from build123d import *

# Parameters (mm, degrees)
CROQUIS1_R              = 1.5
SALIENTE_EXTRUIR1_DEPTH = 3
CROQUIS2_W              = 31.2
CROQUIS2_H              = 31.2
CROQUIS2_W_2            = 28.2
CROQUIS2_H_2            = 28.2
SALIENTE_EXTRUIR2_DEPTH = 9.5
CROQUIS4_W              = 28.2
CROQUIS4_H              = 28.2
CROQUIS4_W_2            = 26.2
CROQUIS4_H_2            = 26.2
SALIENTE_EXTRUIR3_DEPTH = 3
CORTAR_EXTRUIR1_REACH   = 69.732
CROQUIS8_W              = 7.2
CROQUIS8_H              = 1
CORTAR_EXTRUIR2_START   = -9.5
CROQUIS9_W              = 5.627722912
CROQUIS9_H              = 14.2
CORTAR_EXTRUIR2_DEPTH   = 9.5
CROQUIS10_W             = 2.5
CROQUIS10_H             = 31.2
SALIENTE_EXTRUIR4_DEPTH = 1


with BuildPart() as part:
    # Croquis1 → Saliente-Extruir1 (new body)
    with BuildSketch(Plane.XY):
        with BuildLine():
            Line((-52.197309417, 4.461883408), (-50.197309417, 4.461883408))
            Line((-50.197309417, 4.461883408), (-44.197309417, 8.461883408))
            Line((-44.197309417, 8.461883408), (-44.197309417, 24.461883408))
            Line((-44.197309417, 24.461883408), (-50.197309417, 28.461883408))
            Line((-50.197309417, 28.461883408), (-52.197309417, 28.461883408))
            ThreePointArc((-52.197309417, 28.461883408), (-56.197309417, 32.461883408), (-52.197309417, 36.461883408))
            Line((-52.197309417, 36.461883408), (-5.197309417, 36.461883408))
            ThreePointArc((-5.197309417, 36.461883408), (-3.075989073, 35.583203752), (-2.197309417, 33.461883408))
            Line((-2.197309417, 33.461883408), (-2.197309417, 26.567434684))
            ThreePointArc((-2.197309417, 26.567434684), (-2.552285621, 25.151860907), (-3.533208828, 24.071283801))
            Line((-3.533208828, 24.071283801), (-7.361410006, 21.519149682))
            ThreePointArc((-7.361410006, 21.519149682), (-8.342333213, 20.438572576), (-8.697309417, 19.022998799))
            Line((-8.697309417, 19.022998799), (-8.697309417, 13.900768017))
            ThreePointArc((-8.697309417, 13.900768017), (-8.342333213, 12.48519424), (-7.361410006, 11.404617134))
            Line((-7.361410006, 11.404617134), (-3.533208828, 8.852483016))
            ThreePointArc((-3.533208828, 8.852483016), (-2.552285621, 7.771905909), (-2.197309417, 6.356332133))
            Line((-2.197309417, 6.356332133), (-2.197309417, -0.538116592))
            ThreePointArc((-2.197309417, -0.538116592), (-3.075989073, -2.659436935), (-5.197309417, -3.538116592))
            Line((-5.197309417, -3.538116592), (-52.197309417, -3.538116592))
            ThreePointArc((-52.197309417, -3.538116592), (-56.197309417, 0.461883408), (-52.197309417, 4.461883408))
        make_face()
        with Locations((-6.697309417, 32.461883408)):
            Circle(CROQUIS1_R, mode=Mode.SUBTRACT)
        with Locations((-52.197309417, 0.461883408)):
            Circle(CROQUIS1_R, mode=Mode.SUBTRACT)
        with Locations((-6.697309417, 0.461883408)):
            Circle(CROQUIS1_R, mode=Mode.SUBTRACT)
        with Locations((-52.197309417, 32.461883408)):
            Circle(CROQUIS1_R, mode=Mode.SUBTRACT)
    extrude(amount=SALIENTE_EXTRUIR1_DEPTH)

    # Croquis2 → Saliente-Extruir2 (add)
    with BuildSketch(Plane.XY.offset(3)):
        with Locations((-25.447309417, 16.261883408)):
            Rectangle(CROQUIS2_W, CROQUIS2_H)
        with Locations((-25.447309417, 16.261883408)):
            Rectangle(CROQUIS2_W_2, CROQUIS2_H_2, mode=Mode.SUBTRACT)
    extrude(amount=SALIENTE_EXTRUIR2_DEPTH)

    # Croquis4 → Saliente-Extruir3 (add)
    with BuildSketch(Plane.XY.offset(7)):
        with Locations((-25.447309417, 16.261883408)):
            Rectangle(CROQUIS4_W, CROQUIS4_H)
        with Locations((-25.447309417, 16.261883408)):
            Rectangle(CROQUIS4_W_2, CROQUIS4_H_2, mode=Mode.SUBTRACT)
    extrude(amount=SALIENTE_EXTRUIR3_DEPTH)

    # Cortar-Barrer1: sweep along a path in Croquis7
    with BuildLine(Plane.XY.offset(10)) as cortar_barrer1_path:
        Line((-39.047309417, 29.861883408), (-11.847309417, 29.861883408))
        Line((-11.847309417, 29.861883408), (-11.847309417, 2.661883408))
        Line((-11.847309417, 2.661883408), (-39.047309417, 2.661883408))
        Line((-39.047309417, 2.661883408), (-39.047309417, 29.861883408))
    # Croquis6 → Cortar-Barrer1 (sweep, cut)
    with BuildSketch(Plane(origin=(0, 3.161883408, 0), x_dir=(-1, 0, 0), z_dir=(0, -1, 0))):
        Polygon((38.547309417, -8.5), (38.547309417, -7), (39.547309417, -7), align=None)
    sweep(path=cortar_barrer1_path.line, transition=Transition.RIGHT, mode=Mode.SUBTRACT)

    # Cortar-Extruir1: up to this plane
    cortar_extruir1_end = Plane(origin=(-39.697309417, 30.361883408, 7), z_dir=(0, -0.8320502943378436, -0.5547001962252293))
    # Croquis8 → Cortar-Extruir1 (cut, up to the surface)
    with BuildSketch(Plane.XY.offset(10), mode=Mode.PRIVATE) as cortar_extruir1_sk1:
        with Locations((-26.947309417, 29.861883408)):
            Rectangle(CROQUIS8_W, CROQUIS8_H)
    cortar_extruir1_tool1 = split(extrude(cortar_extruir1_sk1.sketch, amount=-CORTAR_EXTRUIR1_REACH, mode=Mode.PRIVATE), bisect_by=cortar_extruir1_end, keep=Keep.BOTH, mode=Mode.PRIVATE)
    add(cortar_extruir1_tool1.solids().sort_by_distance((-26.947309, 29.861883, 10))[0], mode=Mode.SUBTRACT)

    # Croquis9 → Cortar-Extruir2 (cut)
    with BuildSketch(Plane.XY.offset(12.5).offset(CORTAR_EXTRUIR2_START)):
        with Locations((-12.661170873, 16.261883408)):
            Rectangle(CROQUIS9_W, CROQUIS9_H)
    extrude(amount=CORTAR_EXTRUIR2_DEPTH, mode=Mode.SUBTRACT)

    # Croquis10 → Saliente-Extruir4 (add)
    with BuildSketch(Plane.XY.offset(12.5)):
        with Locations((-39.797309417, 16.261883408)):
            Rectangle(CROQUIS10_W, CROQUIS10_H)
    extrude(amount=SALIENTE_EXTRUIR4_DEPTH)


solid = part.part
Read the model definition and answer for the solid it produces. Units are mm, in the model's axes. A direction names the side the tool comes from. Coordinates: 2 decimals unless noted, no trailing zeros. Loops run counter-clockwise (first coordinate to the right, second up) from the corner with the lowest first, then second, coordinate; pieces in that order, holes last. Notation, with made-up numbers: (-15.5, 78.25) -> (13.5, 78.25) arc R16 ccw to (13.5, 90.25) -> close; hole circle Ø3 at (64, 66). An arc over 180 degrees is marked (long way). Write item = value, one per line. Start each with the question number.
1) The mould has two halves that part along X. Classify faces 1 (the face through (-56.196, 0.374, 1.479)), 2 (the face through (-51.391, 33.727, 1.479)), 3 (the face through (-26, 31.862, 8)), 4 (the face through (-3.099, 35.606, 1.479)): pulls with the +X half, pulls with the -X half, needs draft (parallel to the pull), parting line crosses it, or undercut.
2) For faces 5 (the face through (-25.64, 2.67, 7.76)), 6 (the face through (-9.847, 5, 8)), 7 (the face through (-44.197, 16, 1)), determine the directions among +Z, -Z, +X, -X, +Y, -Y from which every point of the face is accessible in a straight line to the end or side of a thin tool.
3) Given P1, Ø2.5, axis at y = 16.5, z = 1, coming from the +X side; P2, Ø3, axis at y = 28.5, z = 6, coming from the -X side; P3, Ø3, axis at x = -21, z = 10.5, coming from the -Y side, each flat-ended and moving along its own axis, determine where each tip first touches the part or whether it passes through.
4) Find the intervals of material crossed by L1, parallel to X at y = 32.5, z = 2; L2, parallel to X at y = 26.5, z = 5; L3, parallel to Y at x = -6, z = 2.75, in increasing order. Write a range as from..to.
5) The part is cut by section A-A, the plane z = 6. Determine the outline of the cut face in (x, y), plus the area to 3 significant figures.
6) The part is cut by section D-D, the plane y = 26. Determine the outline of the cut face in (x, z).
7) The part is cut by section C-C, the plane z = 2.25. Determine the outline of the cut face in (x, y), plus the area to 3 significant figures.
8) The part is cut by section B-B, the plane x = -14. Determine the outline of the cut face in (y, z), plus the area to 3 significant figures.
Result:
q1.face_1 = pulls with the -X half
q1.face_2 = undercut
q1.face_3 = needs draft
q1.face_4 = pulls with the +X half
q2.face_5 = none
q2.face_6 = +Z, +X, +Y, -Y
q2.face_7 = +Z, -Z, -X
q3.P1 = -8.7
q3.P2 = -41.05
q3.P3 = 0.66
q4.L1 = -56.2..-53.7, -50.7..-8.2, -5.2..-2.2
q4.L2 = -41.05..-39.55, -11.35..-9.85
q4.L3 = -3.54..-0.87, 1.79..10.5, 22.43..31.13, 33.79..36.46
q5.outline = (-41.05, 0.66) -> (-9.85, 0.66) -> (-9.85, 9.16) -> (-11.35, 9.16) -> (-11.35, 2.16) -> (-39.55, 2.16) -> (-39.55, 30.36) -> (-11.35, 30.36) -> (-11.35, 23.36) -> (-9.85, 23.36) -> (-9.85, 31.86) -> (-41.05, 31.86) -> close
q5.area = 157 mm²
q6.outline = (-46.5, 0) -> (-2.25, 0) -> (-2.25, 3) -> (-9.85, 3) -> (-9.85, 12.5) -> (-11.35, 12.5) -> (-11.35, 10) -> (-12.35, 10) -> (-12.35, 8.5) -> (-11.35, 7) -> (-11.35, 3) -> (-39.55, 3) -> (-39.55, 7) -> (-38.55, 8.5) -> (-38.55, 10) -> (-39.55, 10) -> (-39.55, 12.5) -> (-38.55, 12.5) -> (-38.55, 13.5) -> (-41.05, 13.5) -> (-41.05, 3) -> (-46.5, 3) -> close
q7.outline = (-52.2, -3.54) -> (-5.2, -3.54) arc R3 ccw to (-2.2, -0.54) -> (-2.2, 6.36) arc R3 ccw to (-3.53, 8.85) -> (-7.36, 11.4) arc R3 cw to (-8.7, 13.9) -> (-8.7, 19.02) arc R3 cw to (-7.36, 21.52) -> (-3.53, 24.07) arc R3 ccw to (-2.2, 26.57) -> (-2.2, 33.46) arc R3 ccw to (-5.2, 36.46) -> (-52.2, 36.46) arc R4 ccw to (-52.2, 28.46) -> (-50.2, 28.46) -> (-44.2, 24.46) -> (-44.2, 8.46) -> (-50.2, 4.46) -> (-52.2, 4.46) arc R4 ccw to start; hole circle Ø3 at (-52.2, 0.46); hole circle Ø3 at (-52.2, 32.46); hole circle Ø3 at (-6.7, 0.46); hole circle Ø3 at (-6.7, 32.46)
q7.area = 1,770 mm²
q8.outline = (-3.54, 0) -> (36.46, 0) -> (36.46, 3) -> (31.86, 3) -> (31.86, 12.5) -> (30.36, 12.5) -> (30.36, 10) -> (29.36, 10) -> (29.36, 8.5) -> (30.36, 7) -> (30.36, 3) -> (2.16, 3) -> (2.16, 7) -> (3.16, 8.5) -> (3.16, 10) -> (2.16, 10) -> (2.16, 12.5) -> (0.66, 12.5) -> (0.66, 3) -> (-3.54, 3) -> close
q8.area = 153 mm²
